Here's how the part is built. I have some questions about the finished solid (model axes, mm). Face numbers are marked on the shaded views. A direction names the side the tool comes from. Give positions to 0.01 mm unless a question says otherwise; leave off trailing zeros. Order: outer loops, then holes, each group sorted by start corner. A loop starts at its lowest first (then second) coordinate and runs counter-clockwise, first axis right, second up. Notation, with made-up numbers: M -38,81 L -7,81 A16 ccw -7,94 Z; hole C -36,36 d8. An arc over 180 degrees is marked long. Use one line per item in the form item = value.
from build123d import *

# Parameters (mm, degrees)
PAD005_DEPTH    = 26.4
SKETCH068_W     = 6
SKETCH068_H     = 40
PAD006_DEPTH    = 13.6
SKETCH070_R     = 1.5
POCKET004_DEPTH = 6
PAD007_DEPTH    = 10
SKETCH071_R     = 1.5
POCKET005_DEPTH = 9
CHAMFER003_SIZE = 12


with BuildPart() as part:
    # Sketch067 → Pad005 (new body)
    with BuildSketch(Plane.XY.offset(19.5)):
        with BuildLine():
            ThreePointArc((0, -11.2), (11.2, 0), (0, 11.2))
            Line((0, 11.2), (0, 14.2))
            Line((0, 14.2), (24, 14.2))
            Line((24, 14.2), (24, 20))
            Line((30, 20), (24, 20))
            Line((30, 20), (30, -20))
            Line((30, -20), (24, -20))
            Line((24, -14.2), (24, -20))
            Line((0, -14.2), (24, -14.2))
            Line((0, -11.2), (0, -14.2))
        make_face()
    extrude(amount=PAD005_DEPTH)

    # Sketch068 → Pad006 (new body)
    with BuildSketch(Plane(origin=(0, 0, 19.5), x_dir=(1, 0, 0), z_dir=(0, 0, -1))):
        with Locations((27, 0)):
            Rectangle(SKETCH068_W, SKETCH068_H)
    extrude(amount=PAD006_DEPTH)

    # Sketch070 → Pocket004 (cut)
    with BuildSketch(Plane(origin=(30, 0, 19.5), x_dir=(0, 1, 0), z_dir=(1, 0, 0))):
        with Locations((-16, 22.4)):
            Circle(SKETCH070_R)
        with Locations((16, 22.4)):
            Circle(SKETCH070_R)
        with Locations((16, -9.6)):
            Circle(SKETCH070_R)
        with Locations((-16, -9.6)):
            Circle(SKETCH070_R)
    extrude(amount=-POCKET004_DEPTH, mode=Mode.SUBTRACT)

    # Sketch069 → Pad007 (new body)
    with BuildSketch(Plane(origin=(0, 0, 19.5), x_dir=(0, -1, 0), z_dir=(-1, 0, 0))):
        with BuildLine():
            ThreePointArc((-11.2, 17.969696), (-17.7, 13.2), (-11.2, 8.430304))
            Line((-11.2, 17.969696), (-11.2, 8.430304))
        make_face()
        with BuildLine():
            ThreePointArc((11.2, 8.430304), (17.7, 13.2), (11.2, 17.969696))
            Line((11.2, 17.969696), (11.2, 8.430304))
        make_face()
    extrude(amount=-PAD007_DEPTH)

    # Sketch071 → Pocket005 (cut)
    with BuildSketch(Plane(origin=(0, 0, 19.5), x_dir=(0, -1, 0), z_dir=(-1, 0, 0))):
        with Locations((-14.2, 13.2)):
            Circle(SKETCH071_R)
        with Locations((14.2, 13.2)):
            Circle(SKETCH071_R)
    extrude(amount=-POCKET005_DEPTH, mode=Mode.SUBTRACT)

    # Chamfer003
    chamfer003_edges = [part.edges().sort_by_distance(p)[0] for p in [
        (24, 0, 19.5),
    ]]
    chamfer(chamfer003_edges, length=CHAMFER003_SIZE)


solid = part.part
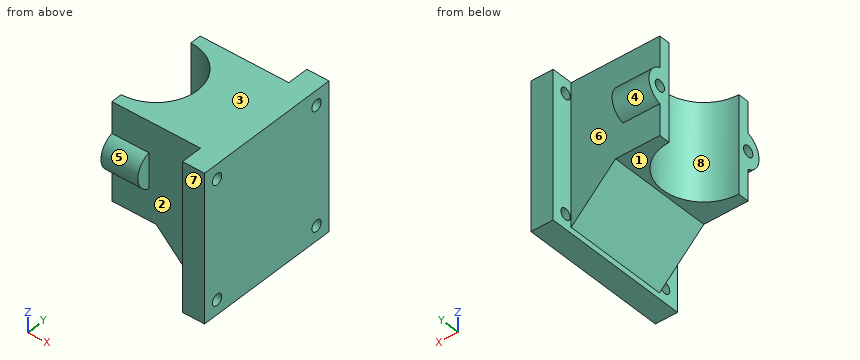
Q1. I need wall thicknesses on L1, parallel to Z at x = 26.4, y = -16; L2, parallel to Y at x = 24.25, z = 42.5; L3, parallel to X at y = -15, z = 25. Which ranges of each line are inside material? Lowest first, please.
Found:
L1 = 5.9 to 8.4, 11.4 to 40.4, 43.4 to 45.9
L2 = -20 to -17.37, -14.63 to 14.63, 17.37 to 20
L3 = 24 to 30
Q2. I want a section at B-B on x = 6. Write out the boundary of the cut face in (y, z), then the cut area to 3 significant figures.
Found:
outline = M -14.2,19.5 L -9.46,19.5 L -9.46,45.9 L -14.2,45.9 L -14.2,37.47 A5 ccw -14.2,27.93 Z; M 9.46,19.5 L 14.2,19.5 L 14.2,27.93 A5 ccw 14.2,37.47 L 14.2,45.9 L 9.46,45.9 Z; hole C -14.2,32.7 d3; hole C 14.2,32.7 d3
area = 285 mm²
Q3. I want a section at C-C on z = 32.7. Write out the boundary of the cut face in (x, y).
Found:
outline = M 0,-17.7 L 10,-17.7 L 10,-14.2 L 24,-14.2 L 24,-20 L 30,-20 L 30,20 L 24,20 L 24,14.2 L 10,14.2 L 10,17.7 L 0,17.7 L 0,15.7 L 9,15.7 L 9,12.7 L 0,12.7 L 0,11.2 A11.2 cw 0,-11.2 L 0,-12.7 L 9,-12.7 L 9,-15.7 L 0,-15.7 Z
Q4. I want a section at D-D on x = 25. Write out the boundary of the cut face in (y, z), then the cut area to 3 significant figures.
Found:
outline = M -20,5.9 L 20,5.9 L 20,45.9 L -20,45.9 Z; hole C -16,9.9 d3; hole C -16,41.9 d3; hole C 16,9.9 d3; hole C 16,41.9 d3
area = 1,570 mm²
Q5. I'm going to push flat-ended pins straight in: pin 1 Ø1.5 at (y, z) = (2, 10.5) entering from -X; pin 2 Ø4 at (y, z) = (16, 9.9) entering from -X; pin 3 Ø6 at (x, z) = (7, 39) entering from -Y; pin 4 Ø3.5 at (y, z) = (-16, 41.9) entering from +X. Where does each tip first touch, or does it pass through?
Found:
pin_1 = 20.25
pin_2 = 20.73
pin_3 = -16.46
pin_4 = 30
Q6. I want a section at A-A on z = 41.9. Write out the boundary of the cut face in (x, y).
Found:
outline = M 0,-14.2 L 24,-14.2 L 24,-14.5 L 30,-14.5 L 30,14.5 L 24,14.5 L 24,14.2 L 0,14.2 L 0,11.2 A11.2 cw 0,-11.2 Z; M 24,-20 L 30,-20 L 30,-17.5 L 24,-17.5 Z; M 24,17.5 L 30,17.5 L 30,20 L 24,20 Z
Q7. On a 3-axis mill with a long thin cutter (end or side, diameter ignored), from which of +Z, -Z, +X, -X, +Y, -Y can I reach the whole of each face in a straight line? I mean the marked faces 1, 2, 3, 4 and 5. Say none if no direction works.
Found:
face_1 = -Z, -X, +Y, -Y
face_2 = -Y
face_3 = +Z, +X, -X, +Y, -Y
face_4 = -X, +Y
face_5 = -X, -Y
Q8. Thinking about a two-plate mould opening in X: for the marked faces 6, 7 and 8, which applies, +X half, -X half, draft (parallel to the pull), parting line (faces both ways), or undercut?
Found:
face_6 = undercut
face_7 = draft
face_8 = -X half
